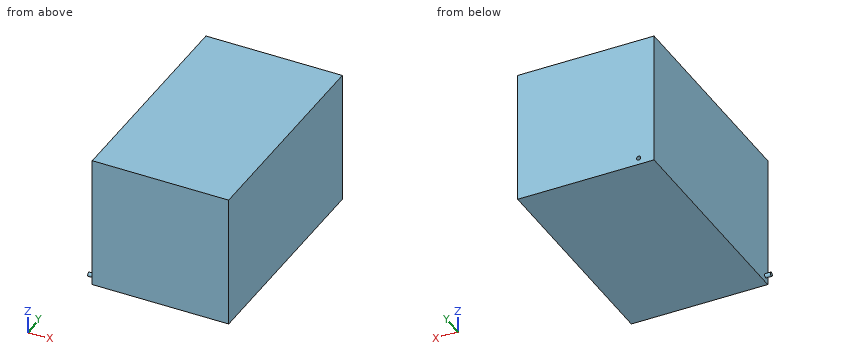
from build123d import *

# Parameters (mm, degrees)
F0_W      = 82.4321992695
F0_H      = 43.8606161624
F1_DEPTH  = 431.8
F2_DEPTH  = 54.864
F3_R      = 7.0871309168
F4_DEPTH  = 20.574
F5_R      = 7.362788809
F6_DEPTH  = 14.478
F7_DEPTH  = 34.544
F8_DEPTH  = 37.084
F9_DEPTH  = 673.1
F10_DEPTH = 431.8


with BuildPart() as f1:
    # F0 (on Right) → F1 (new body)
    with BuildSketch(Plane.YZ):
        with Locations((-5.2245799452, 3.5912198946)):
            Rectangle(F0_W, F0_H)
    extrude(amount=F1_DEPTH)

    # F2 (add): a face of the model
    f2_faces = [f1.faces().sort_by_distance(p)[0] for p in [
        (0, -5.2245799452, 3.5912198946),
    ]]
    extrude(f2_faces, amount=F2_DEPTH)

    # F3 (on face) → F4 (join)
    with BuildSketch(Plane(origin=(-54.864, 0, 0), x_dir=(0, -1, 0), z_dir=(-1, 0, 0))):
        with Locations((31.2521867454, 5.9642316774)):
            Circle(F3_R)
    extrude(amount=F4_DEPTH)

    # F5 (on face) → F6 (join)
    with BuildSketch(Plane(origin=(0, 35.9915196896, 0), x_dir=(-1, 0, 0), z_dir=(0, 1, 0))):
        with Locations((0, 5.1426673308)):
            Circle(F5_R)
    extrude(amount=F6_DEPTH)

    # F7 (add): a face of the model
    f7_faces = [f1.faces().sort_by_distance(p)[0] for p in [
        (189.9838185674, 35.9915196896, 3.5787418462),
    ]]
    extrude(f7_faces, amount=F7_DEPTH)

    # F8 (add): a face of the model
    f8_faces = [f1.faces().sort_by_distance(p)[0] for p in [
        (0, 50.4695196896, 5.1426673308),
    ]]
    extrude(f8_faces, amount=F8_DEPTH)

    # F9 (add): a face of the model
    f9_faces = [f1.faces().sort_by_distance(p)[0] for p in [
        (189.9838185674, 70.5355196896, 3.5787418462),
    ]]
    extrude(f9_faces, amount=F9_DEPTH)

    # F10 (add): a face of the model
    f10_faces = [f1.faces().sort_by_distance(p)[0] for p in [
        (188.468, 348.5974200548, 25.5215279758),
    ]]
    extrude(f10_faces, amount=F10_DEPTH)


solid = f1.part
Can you work these out from the model? Positions are in its coordinate system, mm. Coordinates: 2 decimals unless noted, no trailing zeros. Write each loop counter-clockwise with the first axis right and the second up, starting at its lowest first coordinate (ties: lowest second). Pieces come first, ordered by that corner, then holes. Notation, with made-up numbers: M -21,19 L 28,19 A15 cw 28,25 Z; hole C 88.25,3.25 d10. An arc over 180 degrees is marked long. Use one line per item in the form item = value.
Q1. For P1, Ø1, axis at y = 230, z = 66.5, coming from the -X side; P2, Ø4.5, axis at x = -3.5, z = 3, coming from the +Y side, each with a flat end and sliding along its axis, tell me the tip position at first contact or that it passes through.
Model answer:
P1 = -54.86
P2 = 87.55
Q2. If we section it at B-B (z = 394): Write out the boundary of the cut face in (x, y).
Model answer:
outline = M -54.86,-46.44 L 431.8,-46.44 L 431.8,743.64 L -54.86,743.64 Z
Q3. If we section it at C-C (y = 26): Write out the boundary of the cut face in (x, z).
Model answer:
outline = M -54.86,-18.34 L 431.8,-18.34 L 431.8,457.32 L -54.86,457.32 Z
Q4. If we section it at A-A (y = 563.5): Write out the boundary of the cut face in (x, z).
Model answer:
outline = M -54.86,-18.34 L 431.8,-18.34 L 431.8,457.32 L -54.86,457.32 Z; hole C 0,5.14 d14.73
Q5. I need wall thicknesses on line 1 along Z through (x, y) = (0, 428); line 2 along X through (y, z) = (-4.5, 265). Which ranges of each line are inside material? Lowest first, please. Write a range as from..to.
Model answer:
line_1 = -18.34..-2.22, 12.51..457.32
line_2 = -54.86..431.8
